```python
from build123d import *

# Parameters (mm, degrees)
SKETCH1_W           = 60
SKETCH1_H           = 60
BOSS_EXTRUDE1_DEPTH = 60
CUT_EXTRUDE1_DEPTH  = 60
CUT_EXTRUDE2_DEPTH  = 60
CUT_EXTRUDE3_DEPTH  = 60
CUT_EXTRUDE6_DEPTH  = 60


with BuildPart() as part:
    # Sketch1 → Boss-Extrude1 (new body)
    with BuildSketch(Plane.XY):
        with Locations((30, 30)):
            Rectangle(SKETCH1_W, SKETCH1_H)
    extrude(amount=BOSS_EXTRUDE1_DEPTH)

    # Sketch2 → Cut-Extrude1 (cut)
    with BuildSketch(Plane.XY.offset(60)):
        with BuildLine():
            ThreePointArc((0, 30), (8.786796564, 51.213203436), (30, 60))
            Line((30, 60), (0, 60))
            Line((0, 60), (0, 30))
        make_face()
        with BuildLine():
            ThreePointArc((30, 0), (8.786796564, 8.786796564), (0, 30))
            Line((0, 30), (0, 0))
            Line((0, 0), (30, 0))
        make_face()
    extrude(amount=-CUT_EXTRUDE1_DEPTH, mode=Mode.SUBTRACT)

    # Sketch3 → Cut-Extrude2 (cut)
    with BuildSketch(Plane(origin=(0, 60, 0), x_dir=(1, 0, 0), z_dir=(0, 1, 0))):
        with BuildLine():
            ThreePointArc((0, -29.999999939), (8.786796586, -8.786796543), (30, 0))
            Line((30, 0), (0, 0))
            Line((0, 0), (0, -29.999999939))
        make_face()
        with BuildLine():
            Line((0, -60), (30, -60))
            ThreePointArc((30, -60), (8.786796543, -51.213203414), (0, -29.999999939))
            Line((0, -29.999999939), (0, -60))
        make_face()
    extrude(amount=-CUT_EXTRUDE2_DEPTH, mode=Mode.SUBTRACT)

    # Sketch4 → Cut-Extrude3 (cut)
    with BuildSketch(Plane(origin=(0, 0, 0), x_dir=(0, 0, -1), z_dir=(1, 0, 0))):
        Polygon((0, 60), (-60, 60), (-60, 0), align=None)
    extrude(amount=CUT_EXTRUDE3_DEPTH, mode=Mode.SUBTRACT)

    # Sketch6 → Cut-Extrude6 (cut)
    with BuildSketch(Plane(origin=(0, 60, 0), x_dir=(1, 0, 0), z_dir=(0, 1, 0))):
        with BuildLine():
            Line((15, -15), (15, -45))
            Line((15, -45), (30, -45))
            ThreePointArc((30, -45), (45, -30), (30, -15))
            Line((30, -15), (15, -15))
        make_face()
    extrude(amount=-CUT_EXTRUDE6_DEPTH, mode=Mode.SUBTRACT)


solid = part.part
```
Geometry: final body of the model. Coordinates: model frame, mm. A direction names the side the tool comes from. Round coordinates to 2 decimals unless told otherwise and drop trailing zeros. Write each loop counter-clockwise with the first axis right and the second up, starting at its lowest first coordinate (ties: lowest second). Pieces come first, ordered by that corner, then holes.
Item 1: Section query A-A (x = 42). Return loops of the section in (y, z), plus the area to 3 significant figures.
Item 2: Section query C-C (y = 18.5). Return loops of the section in (x, z), plus the area to 3 significant figures.
Item 3: Pin query (flat end, axial travel): P1, Ø12, axis at x = 31.5, y = 25, coming from the +Z side; P2, Ø8, axis at y = 7.5, z = 13.5, coming from the -X side; P3, Ø1.5, axis at x = 43.5, y = 42, coming from the +Z side. Return the tip coordinate at first contact, or that it passes through.
Item 4: Section query D-D (x = 29). Return loops of the section in (y, z).
Item 5: Set-up query: faces 5 (the face through (23, 23, 15)), 6 (the face through (60, 23, 23)). Return all of +Z, -Z, +X, -X, +Y, -Y with unobstructed straight access to the full face (end or side cutting, diameter ignored); none if empty.
Item 6: Mould query, pull axis Z, two halves, no side actions, for faces 1 (the face through (48, 0, 30)), 2 (the face through (22, 8, 45)), 3 (the face through (50, 30, 30)), 4 (the face through (12.52, 30.42, 5.62)). Classes: +Z half, -Z half, draft (parallel to the pull), parting line (faces both ways), or undercut.
Item 7: Section query B-B (z = 20.5). Return loops of the section in (x, y), plus the area to 3 significant figures.
Item 8: Material intervals for L1, parallel to X at y = 26, z = 30; L2, parallel to X at y = 18, z = 29; L3, parallel to Z at x = 33, y = 34.5, sorted ascending.
Completed:
1. outline: (0, 0) - (60, 0) - (39, 21) - (0, 21) - close; (0, 39) - (21, 39) - (0, 60) - close
1. area: 1,260 mm2
2. outline: (2.29, 18.5) arc R30 ccw to (30, 0) - (60, 0) - (60, 41.5) - (39.63, 41.5) arc R15 cw to (30, 15) - (15, 15) - (15, 41.5) - (2.29, 41.5) - close
2. area: 1,520 mm2
3. P1: stops at z = 17.01
3. P2: stops at x = 6.38
3. P3: stops at z = 18.75
4. outline: (0.02, 0.02) - (59.98, 0.02) - (45, 15) - (0.02, 15) - close; (0.02, 45) - (15, 45) - (0.02, 59.98) - close
5. face 5: +Y, -Y
5. face 6: +Z, -Z, +X, +Y, -Y
6. face 1: draft
6. face 2: undercut
6. face 3: +Z half
6. face 4: -Z half
7. outline: (1.54, 20.5) arc R30 ccw to (15, 4.02) - (15, 39.5) - (1.54, 39.5) - close; (41.61, 0) - (60, 0) - (60, 39.5) - (41.61, 39.5) - close
7. area: 1,120 mm2
8. L1: x = 0.27 to 15, 45 to 60
8. L2: x = 2.5 to 15, 44.97 to 60
8. L3: z = 0 to 15.3
